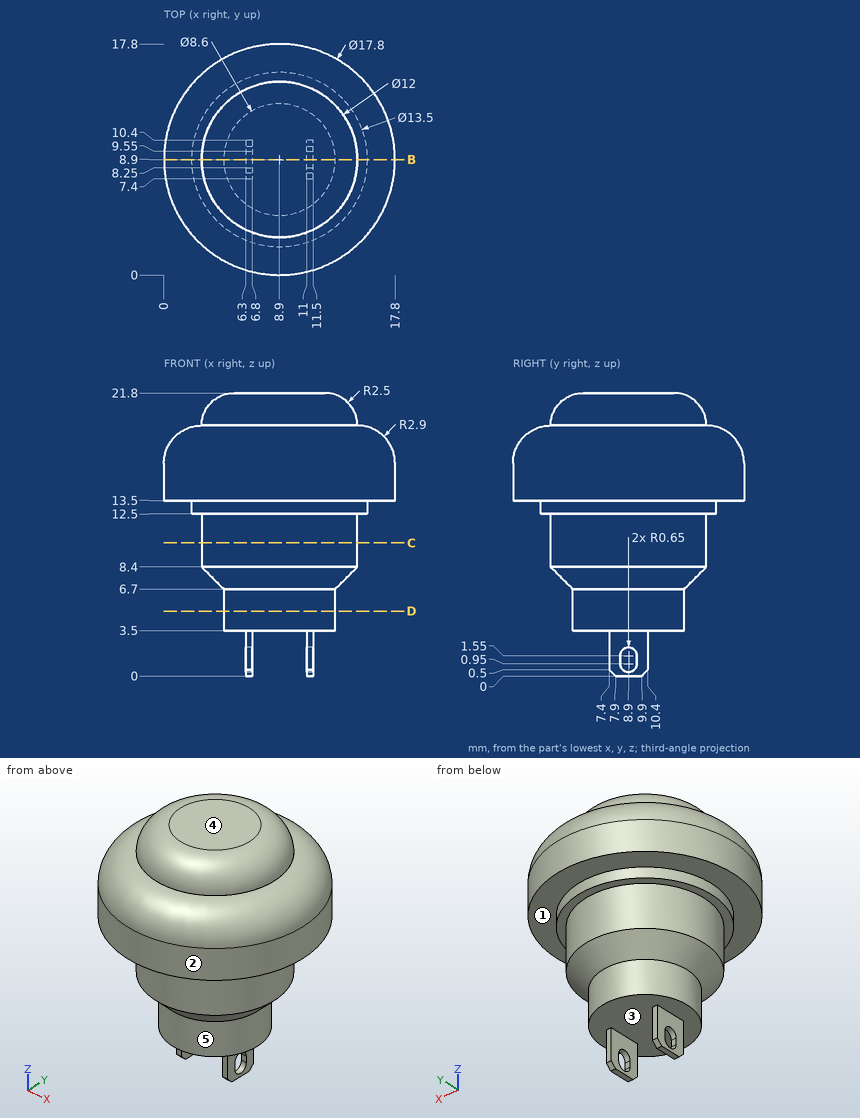
Answer from the drawing. Dimensions are ordinates in mm from the lowest x, y and z of the part. A direction names the side the tool comes from. Give positions to 0.01 mm unless a question says otherwise; leave off trailing zeros. Write each loop counter-clockwise with the first axis right and the second up, starting at its lowest first coordinate (ties: lowest second). Pieces come first, ordered by that corner, then holes.
1) Section C-C (z = 10.25) is taken. Write down the section's boundary in (x, y), and give its area (3 significant figures).
2) Given P1, Ø4.5, axis at x = 10.5, y = 8.5, coming from the -Z side; P2, Ø4, axis at x = 5, z = 18.5, coming from the -Y side; P3, Ø0.6, axis at x = 11, z = 1.5, coming from the +Y side; P4, Ø3, axis at y = 7, z = 8, coming from the +X side, each flat-ended and moving along its own axis, determine where each tip first touches the part or whether it passes through.
3) Section D-D (z = 5) is taken. Write down the section's boundary in (x, y).
4) For a pull along X with two mould halves and no side action, classify the marked faces 3, 4 and 5 as pulls with the +X half, pulls with the -X half, needs draft (parallel to the pull), parting line crosses it, or undercut.
5) Section B-B (y = 8.9) is taken. Count the separate pieces of the cut face and the enclosed holes in it, and give its area (3 significant figures).
6) A tool of negligible diameter and unlimited length cuts with its end or side. For the marked faces 1 and 2, from which of +Z, -Z, +X, -X, +Y, -Y can it reach the whole face along a straight path? Write none if from no direction.
7) Find the intervals of material crossed by L1, parallel to X at y = 9.5, z = 2.5; L2, parallel to Z at x = 8.5, y = 9.75; L3, parallel to Y at x = 5.25, z = 14.5, in increasing order.
Response:
1. outline: circle Ø12 at (8.9, 8.9)
1. area: 113 mm2
2. P1: stops at z = 0
2. P2: stops at y = 0.44
2. P3: stops at y = 10.4
2. P4: stops at x = 14.88
3. outline: circle Ø8.6 at (8.9, 8.9)
4. face 3: undercut
4. face 4: needs draft
4. face 5: parting line crosses it
5. separate pieces: 3
5. enclosed holes: 0
5. area: 236 mm2
6. face 1: -Z
6. face 2: +Z, -Z
7. L1: x = 6.3 to 6.8, 11 to 11.5
7. L2: z = 3.5 to 21.8
7. L3: y = 0.78 to 17.02
